Read the model definition and answer for the solid it produces. Units are mm, in the model's axes. A direction names the side the tool comes from. Give positions to 0.01 mm unless a question says otherwise; leave off trailing zeros. Order: outer loops, then holes, each group sorted by start corner. A loop starts at its lowest first (then second) coordinate and runs counter-clockwise, first axis right, second up.
Item 1: A cutting plane is placed at D-D (z = 92). Write down the section's boundary in (x, y), plus the area to 3 significant figures.
Item 2: A cutting plane is placed at B-B (z = 50). Write down the section's boundary in (x, y), plus the area to 3 significant figures.
Item 3: Given pin 1 Ø0.9 at (y, z) = (1.5, 31.5) entering from +X; pin 2 Ø1.5 at (y, z) = (1.5, 60.5) entering from -X; pin 3 Ø0.9 at (y, z) = (2, 101.5) entering from -X, each flat-ended and moving along its own axis, determine where each tip first touches the part or whether it passes through.
Item 4: Which of the six approach directions +Z, -Z, +X, -X, +Y, -Y give full straight-line access (tool end or side, diameter ignored) to faces 4 (the face through (-189.677, 1.479, 46.647)), 5 (the face through (-134, 3, 58))?
Item 5: A cutting plane is placed at C-C (x = -205). Write down the section's boundary in (y, z), plus the area to 3 significant figures.
Item 6: Find the intervals of material crossed by line 1 along Z through (x, y) = (-225, 1.7); line 2 along X through (y, z) = (1.4, 52); line 3 along X through (y, z) = (2.5, 53.5), in increasing order.
Item 7: A cutting plane is placed at A-A (x = -55.5). Write down the section's boundary in (y, z), plus the area to 3 significant figures.
Item 8: The mould has two halves that part along Z. Classify faces 1 (the face through (-95.323, 1.479, 47.095)), 2 (the face through (-134, 0, 58)), 3 (the face through (-73.677, 1.479, 46.647)): +Z half, -Z half, draft (parallel to the pull), parting line (faces both ways), or undercut.
Autodesk Inventor part; units mm, degrees
ref_plane "YZ Plane" through (0, 0, 0) normal (1, 0, 0) x (0, 1, 0)
ref_plane "XZ Plane" through (0, 0, 0) normal (0, 1, 0) x (-1, 0, 0)
ref_plane "XY Plane" through (0, 0, 0) normal (0, 0, 1) x (1, 0, 0)
sketch "Sketch1" plane through (0, 0, 0) normal (0, 1, 0) x (-1, 0, 0)
  line L0 (0, 0) -> (271, 0)
  line L1 (271, 0) -> (271, 84)
  line L2 (271, 84) -> (0, 84)
  line L3 (0, 84) -> (0, 0)
  line L4 (135.5, 84) -> (135.5, 0) construction
  line L5 (0, 84) -> (-4, 84)
  line L6 (-4, 84) -> (-4, 72)
  line L7 (-4, 72) -> (0, 72)
  line L8 (0, 72) -> (0, 84)
  line L9 (0, 0) -> (-4, 0)
  line L10 (-4, 0) -> (-4, 12)
  line L11 (-4, 12) -> (0, 12)
  line L12 (0, 12) -> (0, 0)
  line L13 (271, 84) -> (271, 0)
  line L14 (271, 84) -> (275, 84)
  line L15 (275, 84) -> (275, 72)
  line L16 (275, 72) -> (271, 72)
  line L17 (271, 72) -> (271, 84)
  line L18 (271, 0) -> (275, 0)
  line L19 (275, 0) -> (275, 12)
  line L20 (275, 12) -> (271, 12)
  line L21 (271, 12) -> (271, 0)
  line L22 (200.5, 46.871) -> (84.5, 46.871) construction
  circle A0 centre (200.5, 46.871) radius 10.825
  arc A1 (201.5, 64.696) -> (199.5, 64.696) centre (200.5, 64.696) ccw
  line L23 (200.5, 57.696) -> (200.5, 64.696) construction
  line L24 (201.5, 57.696) -> (201.5, 64.696)
  line L25 (199.5, 64.696) -> (199.5, 57.696)
  arc A2 (199.5, 57.696) -> (201.5, 57.696) centre (200.5, 57.696) ccw
  arc A3 (201.5, 36.046) -> (199.5, 36.046) centre (200.5, 36.046) ccw
  line L26 (201.5, 29.046) -> (201.5, 36.046)
  arc A4 (199.5, 29.046) -> (201.5, 29.046) centre (200.5, 29.046) ccw
  line L27 (200.5, 36.046) -> (200.5, 29.046) construction
  line L28 (199.5, 36.046) -> (199.5, 29.046)
  arc A5 (85.5, 36.046) -> (83.5, 36.046) centre (84.5, 36.046) ccw
  arc A6 (83.5, 57.696) -> (85.5, 57.696) centre (84.5, 57.696) ccw
  line L29 (83.5, 64.696) -> (83.5, 57.696)
  line L30 (84.5, 57.696) -> (84.5, 64.696) construction
  line L31 (85.5, 57.696) -> (85.5, 64.696)
  arc A7 (85.5, 64.696) -> (83.5, 64.696) centre (84.5, 64.696) ccw
  circle A8 centre (84.5, 46.871) radius 10.825
  arc A9 (83.5, 29.046) -> (85.5, 29.046) centre (84.5, 29.046) ccw
  line L32 (83.5, 36.046) -> (83.5, 29.046)
  line L33 (84.5, 36.046) -> (84.5, 29.046) construction
  line L34 (85.5, 29.046) -> (85.5, 36.046)
  point P0 (200.5, 61.196)
  point P1 (200.5, 32.546)
  point P2 (84.5, 46.871)
  point P3 (84.5, 61.196)
  point P4 (84.5, 32.546)
  dimension "d0" = 271
  dimension "d1" = 84
  dimension "d2" = 4
  dimension "d3" = 12
  dimension "d4" = 4
  dimension "d5" = 12
  dimension "d11" = 116
  dimension "d13" = 37.129
  dimension "d14" = 84.5
  dimension "d15" = 21.65
  dimension "d16" = 7
  dimension "d17" = 2
  dimension "d18" = 7
  dimension "d19" = 2
  dimension "d20" = 21.65
  dimension "d21" = 7
  dimension "d22" = 2
  dimension "d23" = 7
  dimension "d24" = 2
extrude "Extrusion1" add sketch "Sketch1" along normal blind 3
sketch "Sketch3" plane through (0, 0, 0) normal (0, -1, 0) x (1, 0, 0)
  line L0 (4, 0) -> (-275, 0)
  line L1 (-270, 114) -> (0, 114)
  line L2 (0, 114) -> (0, 84)
  line L3 (0, 84) -> (-270, 84)
  line L4 (-270, 84) -> (-270, 114)
  line L5 (-275, 84) -> (4, 84)
  point P0 (0, 0)
  dimension "d28" = 30
extrude "Extrusion2" add sketch "Sketch3" against normal blind 3
sketch "Sketch2" plane through (0, 0, 0) normal (0, -1, 0) x (1, 0, 0)
  circle A0 centre (-232.5, 81.871) radius 1.5 construction
  arc A1 (-199.5011, 36.0922) -> (-199.5011, 57.6498) centre (-200.5, 46.871) ccw
  circle A2 centre (-251.5, 81.871) radius 1.5 construction
  circle A3 centre (-251.5, 98.371) radius 1.5 construction
  circle A4 centre (-232.5, 98.371) radius 1.5 construction
  line L0 (-251.5, 98.371) -> (-232.5, 98.371) construction
  line L1 (-251.5, 98.371) -> (-251.5, 81.871) construction
  line L2 (-252.5, 98.371) -> (-212.5, 98.371) construction
  line L3 (-252.5, 96.871) -> (-212.5, 96.871)
  line L4 (-212.5, 99.871) -> (-252.5, 99.871)
  arc A5 (-252.5, 99.871) -> (-252.5, 96.871) centre (-252.5, 98.371) ccw
  arc A6 (-212.5, 96.871) -> (-212.5, 99.871) centre (-212.5, 98.371) ccw
  line L5 (-252.5, 81.871) -> (-212.5, 81.871) construction
  line L6 (-252.5, 80.371) -> (-212.5, 80.371)
  line L7 (-212.5, 83.371) -> (-252.5, 83.371)
  arc A7 (-252.5, 83.371) -> (-252.5, 80.371) centre (-252.5, 81.871) ccw
  arc A8 (-212.5, 80.371) -> (-212.5, 83.371) centre (-212.5, 81.871) ccw
  circle A9 centre (-52.5, 81.871) radius 1.5 construction
  arc A10 (-83.5011, 36.0922) -> (-83.5011, 57.6498) centre (-84.5, 46.871) ccw construction
  line L8 (-32.5, 81.871) -> (-72.5, 81.871) construction
  line L9 (-32.5, 83.371) -> (-72.5, 83.371)
  line L10 (-72.5, 80.371) -> (-32.5, 80.371)
  arc A11 (-32.5, 80.371) -> (-32.5, 83.371) centre (-32.5, 81.871) ccw
  arc A12 (-72.5, 83.371) -> (-72.5, 80.371) centre (-72.5, 81.871) ccw
  line L11 (-32.5, 98.371) -> (-72.5, 98.371) construction
  line L12 (-32.5, 99.871) -> (-72.5, 99.871)
  line L13 (-72.5, 96.871) -> (-32.5, 96.871)
  arc A13 (-32.5, 96.871) -> (-32.5, 99.871) centre (-32.5, 98.371) ccw
  arc A14 (-72.5, 99.871) -> (-72.5, 96.871) centre (-72.5, 98.371) ccw
  line L14 (-252.5, 65.371) -> (-212.5, 65.371) construction
  line L15 (-252.5, 63.871) -> (-212.5, 63.871)
  line L16 (-212.5, 66.871) -> (-252.5, 66.871)
  arc A15 (-252.5, 66.871) -> (-252.5, 63.871) centre (-252.5, 65.371) ccw
  arc A16 (-212.5, 63.871) -> (-212.5, 66.871) centre (-212.5, 65.371) ccw
  line L17 (-212.5, 81.871) -> (-212.5, 65.371) construction
  line L18 (-32.5, 65.371) -> (-72.5, 65.371) construction
  line L19 (-32.5, 66.871) -> (-72.5, 66.871)
  line L20 (-72.5, 63.871) -> (-32.5, 63.871)
  arc A17 (-32.5, 63.871) -> (-32.5, 66.871) centre (-32.5, 65.371) ccw
  arc A18 (-72.5, 66.871) -> (-72.5, 63.871) centre (-72.5, 65.371) ccw
  line L21 (-72.5, 81.871) -> (-72.5, 65.371) construction
  line L22 (-72.5, 98.371) -> (-72.5, 81.871) construction
  point P0 (0, 0)
  point P1 (-52.5, 98.371)
  point P2 (-232.5, 65.371)
  point P3 (-52.5, 65.371)
  dimension "d25" = 3
  dimension "d26" = 32
  dimension "d27" = 35
  dimension "d31" = 3
  dimension "d32" = 3
  dimension "d33" = 3
  dimension "d34" = 19
  dimension "d35" = 16.5
  dimension "d38" = 20
  dimension "d39" = 20
  dimension "d40" = 3
  dimension "d41" = 3
  dimension "d43" = 32
  dimension "d44" = 35
  dimension "d45" = 20
  dimension "d46" = 3
  dimension "d47" = 20
  dimension "d48" = 3
  dimension "d49" = 20
  dimension "d50" = 3
  dimension "d51" = 16.5
  dimension "d52" = 20
  dimension "d53" = 3
  dimension "d54" = 16.5
extrude "Extrusion3" cut sketch "Sketch2" against normal blind 3
equation "\"d4\" = d2"
equation "\"d31\" = d25"
equation "\"d32\" = d25"
equation "\"d33\" = d25"
equation "\"d41\" = d40"
equation "\"d43\" = d26"
equation "\"d44\" = d27"
properties part number "flipper-support"
Response values:
1. outline: (-270, 0) - (0, 0) - (0, 3) - (-270, 3) - close
1. area: 810 mm2
2. outline: (-271, 0) - (-210.86, 0) - (-210.86, 3) - (-271, 3) - close; (-190.14, 0) - (-94.86, 0) - (-94.86, 3) - (-190.14, 3) - close; (-74.14, 0) - (0, 0) - (0, 3) - (-74.14, 3) - close
2. area: 689 mm2
3. pin 1: stops at x = 0
3. pin 2: stops at x = -271
3. pin 3: stops at x = -270
4. face 4: +Y, -Y
4. face 5: +Z, -Z, +X, -X, +Y
5. outline: (0, 0) - (3, 0) - (3, 37.03) - (0, 37.03) - close; (0, 56.72) - (3, 56.72) - (3, 114) - (0, 114) - close
5. area: 283 mm2
6. line 1: z = 0 to 63.87, 66.87 to 80.37, 83.37 to 96.87, 99.87 to 114
6. line 2: x = -271 to -210.03, -190.97 to -94.03, -74.97 to 0
6. line 3: x = -271 to -209.06, -191.94 to -93.06, -75.94 to 0
7. outline: (0, 0) - (3, 0) - (3, 63.87) - (0, 63.87) - close; (0, 66.87) - (3, 66.87) - (3, 80.37) - (0, 80.37) - close; (0, 83.37) - (3, 83.37) - (3, 96.87) - (0, 96.87) - close; (0, 99.87) - (3, 99.87) - (3, 114) - (0, 114) - close
7. area: 315 mm2
8. face 1: undercut
8. face 2: draft
8. face 3: undercut
